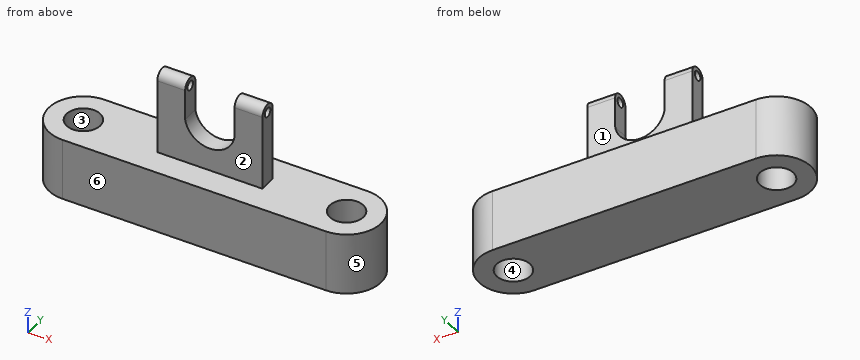
from build123d import *

# Parameters (mm, degrees)
F0_R      = 6.9387858197
F1_DEPTH  = 25.4
F2_W      = 43.0467336029
F2_H      = 6.9942568773
F3_DEPTH  = 5.08
F5_DEPTH  = 6.9942568773
F7_DEPTH  = 11.4016152248
F9_DEPTH  = 11.4016152248
F10_R     = 1.905
F11_DEPTH = 11.4016152248
F12_R     = 1.905
F13_DEPTH = 11.4016152248


with BuildPart() as f1:
    # F0 (on Top) → F1 (new body)
    with BuildSketch(Plane.XY):
        with BuildLine():
            Line((59.8869994283, 10.7242316008), (-47.837305814, 10.7242316008))
            ThreePointArc((-47.837305814, 10.7242316008), (-62.055950053, -3.4944126382), (-47.837305814, -17.7130568773))
            Line((-47.837305814, -17.7130568773), (59.8869994283, -17.7130568773))
            ThreePointArc((59.8869994283, -17.7130568773), (74.1056436673, -3.4944126382), (59.8869994283, 10.7242316008))
        make_face()
        with Locations((-47.837305814, -3.4944126382)):
            Circle(F0_R, mode=Mode.SUBTRACT)
        with Locations((59.8869994283, -3.4944126382)):
            Circle(F0_R, mode=Mode.SUBTRACT)
    extrude(amount=F1_DEPTH)

    # F2 (on face) → F3 (join)
    with BuildSketch(Plane.XY.offset(25.4)):
        with Locations((6.0248468071, -3.4971284386)):
            Rectangle(F2_W, F2_H)
    extrude(amount=F3_DEPTH)

    # F4 (on face) → F5 (join, through all)
    with BuildSketch(Plane(origin=(0, 0, 0), x_dir=(-1, 0, 0), z_dir=(0, 1, 0))):
        with BuildLine():
            Line((-27.5482136086, 56.1515986919), (-27.5482136086, 30.48))
            Line((-27.5482136086, 30.48), (15.4985199943, 30.48))
            Line((15.4985199943, 30.48), (15.4985199943, 56.1515986919))
            Line((15.4985199943, 56.1515986919), (4.0969047695, 56.1515986919))
            Line((4.0969047695, 56.1515986919), (4.0969047695, 43.6199121177))
            ThreePointArc((4.0969047695, 43.6199121177), (-6.0248468071, 34.804850773), (-16.1465983838, 43.6199121177))
            Line((-16.1465983838, 43.6199121177), (-16.1465983838, 56.1515986919))
            Line((-16.1465983838, 56.1515986919), (-27.5482136086, 56.1515986919))
        make_face()
    extrude(amount=-F5_DEPTH)

    # F6 (on face) → F7 (join, through all)
    with BuildSketch(Plane.YZ.offset(27.5482136086)):
        with BuildLine():
            Line((-6.9942568773, 56.1515986919), (0, 56.1515986919))
            ThreePointArc((0, 56.1515986919), (-3.4971284386, 59.6487271306), (-6.9942568773, 56.1515986919))
        make_face()
    extrude(amount=-F7_DEPTH)

    # F8 (on face) → F9 (join, through all)
    with BuildSketch(Plane(origin=(-15.4985199943, 0, 0), x_dir=(0, -1, 0), z_dir=(-1, 0, 0))):
        with BuildLine():
            Line((0, 56.1515986919), (6.9942568773, 56.1515986919))
            ThreePointArc((6.9942568773, 56.1515986919), (3.4971284386, 59.6487271306), (0, 56.1515986919))
        make_face()
    extrude(amount=-F9_DEPTH)

    # F10 (on face) → F11 (cut, through all)
    with BuildSketch(Plane.YZ.offset(27.5482136086)):
        with Locations((-3.4971284386, 56.1515986919)):
            Circle(F10_R)
    extrude(amount=-F11_DEPTH, mode=Mode.SUBTRACT)

    # F12 (on face) → F13 (cut, through all)
    with BuildSketch(Plane(origin=(-15.4985199943, 0, 0), x_dir=(0, -1, 0), z_dir=(-1, 0, 0))):
        with Locations((3.4971284386, 56.1515986919)):
            Circle(F12_R)
    extrude(amount=-F13_DEPTH, mode=Mode.SUBTRACT)


solid = f1.part
For this review, take the finished solid that the model builds, in its own axes (mm). Face numbers are marked on the shaded views. A direction names the side the tool comes from. Round coordinates to 2 decimals unless told otherwise and drop trailing zeros. Loops run counter-clockwise (first coordinate to the right, second up) from the corner with the lowest first, then second, coordinate; pieces in that order, holes last. Notation, with made-up numbers: (-2, 58.5) - (40, 58.5) arc R20 ccw to (40, 66.5) - close; hole circle Ø2 at (-30, 70.5). An arc over 180 degrees is marked (long way). One line per item, written item: value. Start each with the question number.
Item 1: Take a section at D-D (x = -2). Give the boundary of the cut face in (y, z), plus the area to 3 significant figures.
Item 2: Take a section at A-A (z = 48.5). Give the boundary of the cut face in (x, y), plus the area to 3 significant figures.
Item 3: Take a section at C-C (x = -45). Give the boundary of the cut face in (y, z).
Item 4: Clearance check with flat-ended pins moving along their axes: pin 1 Ø6 at (x, y) = (25, -1) entering from -Z; pin 2 Ø2 at (y, z) = (-6.5, 49.5) entering from -X; pin 3 Ø1.5 at (y, z) = (-3, 44.5) entering from +X; pin 4 Ø5 at (x, y) = (-22, -13.5) entering from +Z. State where each tip first meets the part, or that it passes through.
Item 5: The part is to be moulded in two halves that separate along X. For the marked faces 4, 5 and 6, say which applies: +X half, -X half, draft (parallel to the pull), parting line (faces both ways), or undercut.
Item 6: For L1, parallel to X at y = -3.75, z = 8; L2, parallel to X at y = 1, z = 10; L3, parallel to Z at x = -54.5, y = 4.25, list the stretches that pass through material, from the lowest coordinate up.
Item 7: Take a section at B-B (y = 1.75). Give the boundary of the cut face in (x, z).
Item 8: For the marked faces 1, 2 and 3, list the 3-axis set-ups (+Z, -Z, +X, -X, +Y, -Y) from which the entire face can be reached by the end or side of a thin tool; tool diameter is ignored.
Answer below:
1. outline: (-17.71, 0) - (10.72, 0) - (10.72, 25.4) - (0, 25.4) - (0, 38.7) - (-6.99, 38.7) - (-6.99, 25.4) - (-17.71, 25.4) - close
1. area: 815 mm2
2. outline: (-15.5, -6.99) - (-4.1, -6.99) - (-4.1, 0) - (-15.5, 0) - close; (16.15, -6.99) - (27.55, -6.99) - (27.55, 0) - (16.15, 0) - close
2. area: 159 mm2
3. outline: (-17.71, 0) - (-9.83, 0) - (-9.83, 25.4) - (-17.71, 25.4) - close; (2.84, 0) - (10.72, 0) - (10.72, 25.4) - (2.84, 25.4) - close
4. pin 1: stops at z = 0
4. pin 2: stops at x = -15.5
4. pin 3: stops at x = 27.55
4. pin 4: stops at z = 25.4
5. face 4: undercut
5. face 5: +X half
5. face 6: draft
6. L1: x = -62.05 to -54.77, -40.9 to 52.95, 66.82 to 74.1
6. L2: x = -61.33 to -53.12, -42.55 to 54.6, 65.17 to 73.38
6. L3: z = 0 to 25.4
7. outline: (-61.05, 0) - (-52.38, 0) - (-52.38, 25.4) - (-61.05, 25.4) - close; (-43.29, 0) - (55.34, 0) - (55.34, 25.4) - (-43.29, 25.4) - close; (64.43, 0) - (73.1, 0) - (73.1, 25.4) - (64.43, 25.4) - close
8. face 1: +Z, +X, -X, +Y
8. face 2: +Z, +X, -X, -Y
8. face 3: +Z, -Z
